Part model, mm, in its own coordinate system. Coordinates: 2 decimals unless noted, no trailing zeros. Loops run counter-clockwise (first coordinate to the right, second up) from the corner with the lowest first, then second, coordinate; pieces in that order, holes last. Notation, with made-up numbers: M 58,-11.5 L 89,-11.5 A22 ccw 89,22.5 Z; hole C 59.5,64.25 d3. An arc over 180 degrees is marked long. Answer as a JSON object with one key per item and string values. Group by question number.
1. Saw through at D-D on y = 23. Write the cut outline in (x, z).
2. Saw through at B-B on y = 10. Write the cut outline in (x, z), then the cut area to 3 significant figures.
3. Mould opens along X. For faces 1 (the face through (-0.1, 40.5, 1.5)), 2 (the face through (0, 24, 3)), 3 (the face through (2.19, 13.504, 1.479)) say: released by +X, released by -X, zero draft, split by the parting line, or undercut.
4. Drill centre lines: L1, parallel to Y at x = 0, z = 2.1; L2, parallel to Y at x = 1, z = 1.7; L3, parallel to X at y = 6, z = 1.05. Where is each one in solid material? Low to high.
5. Drop flat-ended pins along their axis: pin 1 Ø1.5 at (x, y) = (0, 0) entering from +Z; pin 2 Ø1 at (x, z) = (-2.5, 2.5) entering from +Y; pin 3 Ø1.5 at (x, z) = (1.5, 1.5) entering from +Y. Give the stop position or say it passes through.
6. Saw through at C-C on y = 15. Write the cut outline in (x, z).
Autodesk Inventor part; units mm, degrees
ref_plane "YZ Plane" through (0, 0, 0) normal (1, 0, 0) x (0, 1, 0)
ref_plane "XZ Plane" through (0, 0, 0) normal (0, 1, 0) x (-1, 0, 0)
ref_plane "XY Plane" through (0, 0, 0) normal (0, 0, 1) x (1, 0, 0)
sketch "Boceto1" plane through (0, 0, 0) normal (0, 0, 1) x (1, 0, 0)
  circle A0 centre (0, 0) radius 1.25
  arc A1 (-2.2988, -0.0746) -> (2.2988, -0.0746) centre (0, 0) ccw
  arc A2 (3.4982, 36.8865) -> (-3.4982, 36.8865) centre (0, 37) ccw
  circle A3 centre (0, 37) radius 1.75
  line L0 (0, 0) -> (0, 37) construction
  line L1 (-3.4982, 36.8865) -> (-2.2988, -0.0746)
  line L2 (3.4982, 36.8865) -> (2.2988, -0.0746)
  circle A4 centre (0, 5) radius 1.25
  circle A5 centre (0, 10) radius 1.25
  circle A6 centre (0, 26) radius 1.25
  circle A7 centre (2.2552, 14) radius 0.5
  point P0 (2.755, 13.9838)
  dimension "d0" = 37
  dimension "d1" = 7
  dimension "d2" = 3.5
  dimension "d3" = 4.6
  dimension "d4" = 2.5
  dimension "d5" = 2.5
  dimension "d6" = 2.5
  dimension "d7" = 2.5
  dimension "d8" = 5
  dimension "d9" = 5
  dimension "d10" = 4
  dimension "d11" = 1
  dimension "d12" = 12
extrude "Extrusión1" add sketch "Boceto1" along normal blind 3
equation "\"d5\" = d4"
equation "\"d6\" = d4"
equation "\"d7\" = d4"
properties part number "Hudson 1-65"
Outcome:
{
 "1": {"outline": "M -3.05,0 L 3.05,0 L 3.05,3 L -3.05,3 Z"},
 "2": {"outline": "M -2.63,0 L -1.25,0 L -1.25,3 L -2.63,3 Z; M 1.25,0 L 2.63,0 L 2.63,3 L 1.25,3 Z", "area": "8.25 mm²"},
 "3": {"face 1": "split by the parting line", "face 2": "zero draft", "face 3": "undercut"},
 "4": {"L1": "y = -2.3 to -1.25, 1.25 to 3.75, 6.25 to 8.75, 11.25 to 24.75, 27.25 to 35.25, 38.75 to 40.5", "L2": "y = -2.07 to -0.75, 0.75 to 4.25, 5.75 to 9.25, 10.75 to 25.25, 26.75 to 35.56, 38.44 to 40.35", "L3": "x = -2.5 to -0.75, 0.75 to 2.5"},
 "5": {"pin 1": "passes through", "pin 2": "stops at y = 39.87", "pin 3": "stops at y = 40.42"},
 "6": {"outline": "M -2.79,0 L 2.79,0 L 2.79,3 L -2.79,3 Z"}
}
